CAD build for the part. Positions are in the model's coordinates, mm. Face numbers are marked on the shaded views. Round coordinates to 2 decimals unless told otherwise and drop trailing zeros. Loops run counter-clockwise (first coordinate to the right, second up) from the corner with the lowest first, then second, coordinate; pieces in that order, holes last. Notation, with made-up numbers: M 77.25,81 L 89.25,81 A17 ccw 89.25,100 Z; hole C -5.75,-12.75 d3. An arc over 180 degrees is marked long. One line per item, written item: value. Start each with the question number.
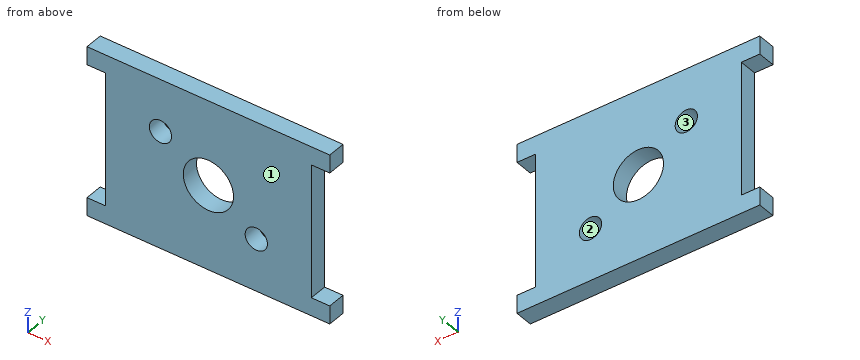
from build123d import *

# Parameters (mm, degrees)
SKETCH1_W           = 39.878
SKETCH1_H           = 27.8384
BOSS_EXTRUDE1_DEPTH = 2.921
CUT_EXTRUDE2_REACH  = 50.721
SKETCH3_W           = 3.0226
SKETCH3_H           = 21.8948
CUT_EXTRUDE1_REACH  = 50.721
SKETCH2_R           = 4.1275
SKETCH2_R_2         = 1.8288


with BuildPart() as part:
    # Sketch1 → Boss-Extrude1 (new body)
    with BuildSketch(Plane(origin=(0, 0, 0), x_dir=(1, 0, 0), z_dir=(0, 1, 0))):
        with Locations((19.939, 13.9192)):
            Rectangle(SKETCH1_W, SKETCH1_H)
    extrude(amount=BOSS_EXTRUDE1_DEPTH)

    # Sketch3 → Cut-Extrude2 (cut, up to next)
    with BuildSketch(Plane(origin=(0, 2.921, 0), x_dir=(1, 0, 0), z_dir=(0, 1, 0)), mode=Mode.PRIVATE) as cut_extrude2_sk1:
        with Locations((1.5113, 13.9192)):
            Rectangle(SKETCH3_W, SKETCH3_H)
    cut_extrude2_tool1 = extrude(cut_extrude2_sk1.sketch, amount=-CUT_EXTRUDE2_REACH, mode=Mode.PRIVATE) & part.part
    # Sketch3 → Cut-Extrude2 (cut, up to next)
    with BuildSketch(Plane(origin=(0, 2.921, 0), x_dir=(1, 0, 0), z_dir=(0, 1, 0)), mode=Mode.PRIVATE) as cut_extrude2_sk2:
        with Locations((38.3667, 13.9192)):
            Rectangle(SKETCH3_W, SKETCH3_H)
    cut_extrude2_tool2 = extrude(cut_extrude2_sk2.sketch, amount=-CUT_EXTRUDE2_REACH, mode=Mode.PRIVATE) & part.part
    add(cut_extrude2_tool1.solids().sort_by_distance((1.5113, 2.921, -13.9192))[0], mode=Mode.SUBTRACT)
    add(cut_extrude2_tool2.solids().sort_by_distance((38.3667, 2.921, -13.9192))[0], mode=Mode.SUBTRACT)

    # Sketch2 → Cut-Extrude1 (cut, up to next)
    with BuildSketch(Plane(origin=(0, 2.921, 0), x_dir=(1, 0, 0), z_dir=(0, 1, 0)), mode=Mode.PRIVATE) as cut_extrude1_sk1:
        with Locations(Location((19.939, 13.9192, 0), (0, 0, 270))):
            Circle(SKETCH2_R)
    cut_extrude1_tool1 = extrude(cut_extrude1_sk1.sketch, amount=-CUT_EXTRUDE1_REACH, mode=Mode.PRIVATE) & part.part
    # Sketch2 → Cut-Extrude1 (cut, up to next)
    with BuildSketch(Plane(origin=(0, 2.921, 0), x_dir=(1, 0, 0), z_dir=(0, 1, 0)), mode=Mode.PRIVATE) as cut_extrude1_sk2:
        with Locations(Location((12.065, 8.5852, 0), (0, 0, 270))):
            Circle(SKETCH2_R_2)
    cut_extrude1_tool2 = extrude(cut_extrude1_sk2.sketch, amount=-CUT_EXTRUDE1_REACH, mode=Mode.PRIVATE) & part.part
    # Sketch2 → Cut-Extrude1 (cut, up to next)
    with BuildSketch(Plane(origin=(0, 2.921, 0), x_dir=(1, 0, 0), z_dir=(0, 1, 0)), mode=Mode.PRIVATE) as cut_extrude1_sk3:
        with Locations(Location((27.813, 19.2532, 0), (0, 0, 270))):
            Circle(SKETCH2_R_2)
    cut_extrude1_tool3 = extrude(cut_extrude1_sk3.sketch, amount=-CUT_EXTRUDE1_REACH, mode=Mode.PRIVATE) & part.part
    add(cut_extrude1_tool1.solids().sort_by_distance((19.939, 2.921, -13.9192))[0], mode=Mode.SUBTRACT)
    add(cut_extrude1_tool2.solids().sort_by_distance((12.065, 2.921, -8.5852))[0], mode=Mode.SUBTRACT)
    add(cut_extrude1_tool3.solids().sort_by_distance((27.813, 2.921, -19.2532))[0], mode=Mode.SUBTRACT)


solid = part.part
(1) Mould opens along Z. For the marked faces 1, 2 and 3 say: pulls with the +Z half, pulls with the -Z half, needs draft (parallel to the pull), parting line crosses it, or undercut.
(2) Slice it at B-B, the plane x = 11.5. List the corners of the cut face in (y, z).
(3) Probe L1, parallel to Z at x = 38.5, y = 1.55; L2, parallel to X at y = 2.45, z = -14; L3, parallel to X at y = 1.95, z = -8.75. List the from-to ranges inside material, lowest first.
(4) Slice it at A-A, the plane z = -8. List the corners of the cut face in (x, y), and give its area (3 significant figures).
(5) Slice it at C-C, the plane y = 2.4. List the corners of the cut face in (x, z) (1 decimal).
(6) Flat gauge pins, fed straight in: P1, Ø0.9, axis at y = 1.5, z = -10.5, coming from the -X side; P2, Ø1, axis at y = 1.5, z = -19, coming from the +X side. Where does each tip first touch, or does it go through?
Check result:
1. face 1: needs draft
1. face 2: undercut
1. face 3: undercut
2. outline: M 0,-27.84 L 2.92,-27.84 L 2.92,-10.32 L 0,-10.32 Z; M 0,-6.85 L 2.92,-6.85 L 2.92,0 L 0,0 Z
3. L1: z = -27.84 to -24.87, -2.97 to 0
3. L2: x = 3.02 to 15.81, 24.07 to 36.86
3. L3: x = 3.02 to 10.24, 13.89 to 36.86
4. outline: M 3.02,0 L 10.33,0 L 10.33,2.92 L 3.02,2.92 Z; M 13.8,0 L 36.86,0 L 36.86,2.92 L 13.8,2.92 Z
4. area: 88.7 mm^2
5. outline: M 0,-27.8 L 39.9,-27.8 L 39.9,-24.9 L 36.9,-24.9 L 36.9,-3 L 39.9,-3 L 39.9,0 L 0,0 L 0,-3 L 3,-3 L 3,-24.9 L 0,-24.9 Z; hole C 12.1,-8.6 d3.7; hole C 19.9,-13.9 d8.3; hole C 27.8,-19.3 d3.7
6. P1: stops at x = 3.02
6. P2: stops at x = 36.86
